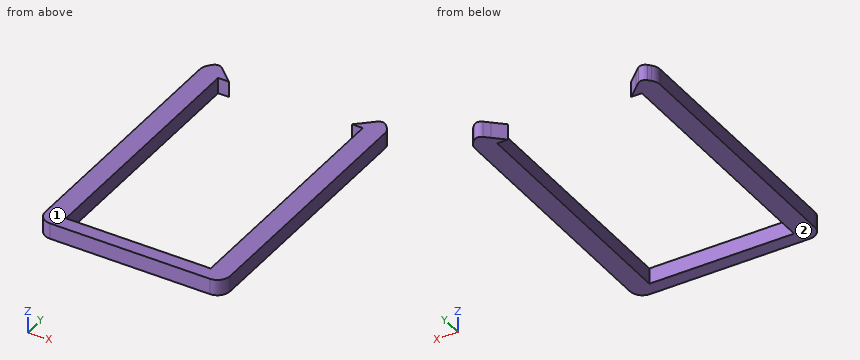
```python
from build123d import *

# Parameters (mm, degrees)
F1_DEPTH = 1.25
F2_R     = 1
F3_R     = 1
F4_R     = 0.5


with BuildPart() as f1:
    # F0 (on Top) → F1 (new body)
    with BuildSketch(Plane.XY):
        Polygon((-7.965586, 11.031977), (-7.965586, -9.196173), (-6.375586, -9.196173), (-6.375586, 10.403827), (-6.375586, 11.178903), (-7.170586, 11.903827), align=None)
        Polygon((-6.375586, 11.178903), (-6.375586, 10.403827), (-5.525586, 10.403827), align=None)
        Polygon((4.194414, 10.403827), (5.044414, 10.403827), (5.044414, 11.178903), align=None)
        Polygon((5.044414, 10.403827), (5.044414, -9.196173), (6.634414, -9.196173), (6.634414, 11.031977), (5.839414, 11.903827), (5.044414, 11.178903), align=None)
        Polygon((-6.375586, -9.196173), (-7.965586, -9.196173), (-7.965586, -10.276173), (6.634414, -10.276173), (6.634414, -9.196173), (5.044414, -9.196173), align=None)
    extrude(amount=F1_DEPTH)

    # F2
    f2_edges = [f1.edges().sort_by_distance(p)[0] for p in [
        (6.634414, -10.276173, 0.625),
        (-7.965586, -10.276173, 0.625),
    ]]
    fillet(f2_edges, radius=F2_R)

    # F3
    f3_edges = [f1.edges().sort_by_distance(p)[0] for p in [
        (-7.965586, 11.031977, 0.625),
        (6.634414, 11.031977, 0.625),
    ]]
    fillet(f3_edges, radius=F3_R)

    # F4
    f4_edges = [f1.edges().sort_by_distance(p)[0] for p in [
        (5.839414, 11.903827, 0.625),
        (-7.170586, 11.903827, 0.625),
    ]]
    fillet(f4_edges, radius=F4_R)


solid = f1.part
```
The model under review builds one solid part; all positions refer to its coordinate system, in mm. Face numbers are marked on the shaded views. Give positions to 0.01 mm unless a question says otherwise; leave off trailing zeros. Write each loop counter-clockwise with the first axis right and the second up, starting at its lowest first coordinate (ties: lowest second). Pieces come first, ordered by that corner, then holes. Notation, with made-up numbers: M 46,-13.75 L 69,-13.75 A21 ccw 69,-2.75 Z; hole C -7.75,-31.5 d8. An arc over 180 degrees is marked long. Answer in a Markdown table with one row per item.
Item 1: Draft analysis for pull direction Z (two halves, no side actions). For the marked faces 1 and 2, state which applies: +Z half, -Z half, draft (parallel to the pull), parting line (faces both ways), or undercut.
Check sheet entries:
| item | result |
|---|---|
| face 1 | +Z half |
| face 2 | -Z half |
Item 2: Add section A-A on z = 0.4. Give the boundary of the cut face in (x, y).
Check sheet entries:
| item | result |
|---|---|
| outline | M -7.97,-9.28 A1 ccw -6.97,-10.28 L 5.63,-10.28 A1 ccw 6.63,-9.28 L 6.63,10.64 A1 ccw 6.37,11.32 L 6.18,11.53 A0.5 ccw 5.47,11.57 L 4.19,10.4 L 5.04,10.4 L 5.04,-9.2 L -6.38,-9.2 L -6.38,10.4 L -5.53,10.4 L -6.8,11.57 A0.5 ccw -7.51,11.53 L -7.7,11.32 A1 ccw -7.97,10.64 Z |
Item 3: Add section B-B on y = -2.5. Give the boundary of the cut face in (x, z).
Check sheet entries:
| item | result |
|---|---|
| outline | M -7.97,0 L -6.38,0 L -6.38,1.25 L -7.97,1.25 Z; M 5.04,0 L 6.63,0 L 6.63,1.25 L 5.04,1.25 Z |
Item 4: For line 1 along X through (y, z) = (-6.5, 0.1); line 2 along Y through (x, z) = (-2.25, 0.65); line 3 along Y through (x, z) = (-6.25, 0.85), list the stretches that pass through material, from the lowest coordinate up.
Check sheet entries:
| item | result |
|---|---|
| line 1 | -7.97 to -6.38, 5.04 to 6.63 |
| line 2 | -10.28 to -9.2 |
| line 3 | -10.28 to -9.2, 10.4 to 11.06 |
Item 5: Add section C-C on x = 4.75. Give the boundary of the cut face in (y, z), plus the area to 3 significant figures.
Check sheet entries:
| item | result |
|---|---|
| outline | M -10.28,0 L -9.2,0 L -9.2,1.25 L -10.28,1.25 Z; M 10.4,0 L 10.91,0 L 10.91,1.25 L 10.4,1.25 Z |
| area | 1.98 mm2 |
Item 6: Add section D-D on x = 0.5. Give the boundary of the cut face in (y, z).
Check sheet entries:
| item | result |
|---|---|
| outline | M -10.28,0 L -9.2,0 L -9.2,1.25 L -10.28,1.25 Z |
